```python
from build123d import *

# Parameters (mm, degrees)
F0_W      = 40
F0_H      = 11
F1_DEPTH  = 10
F2_R      = 8
F3_DEPTH  = 6
F4_R      = 6
F5_DEPTH  = 6
F6_W      = 11
F6_H      = 10
F7_DEPTH  = 2
F8_W      = 11
F8_H      = 10
F9_DEPTH  = 2
F10_R     = 5
F11_R     = 1.75
F12_DEPTH = 25
F13_R     = 2.75
F13_R_2   = 1.75
F14_DEPTH = 2


with BuildPart() as f1:
    # F0 (on Top) → F1 (new body)
    with BuildSketch(Plane.XY):
        with Locations((20, 5.5)):
            Rectangle(F0_W, F0_H)
    extrude(amount=F1_DEPTH)

    # F2 (on face) → F3 (cut)
    with BuildSketch(Plane.XZ):
        with Locations((20, 10)):
            Circle(F2_R)
    extrude(amount=-F3_DEPTH, mode=Mode.SUBTRACT)

    # F4 (on face) → F5 (cut)
    with BuildSketch(Plane(origin=(0, 11, 0), x_dir=(-1, 0, 0), z_dir=(0, 1, 0))):
        with Locations((-20, 10)):
            Circle(F4_R)
    extrude(amount=-F5_DEPTH, mode=Mode.SUBTRACT)

    # F6 (on face) → F7 (join)
    with BuildSketch(Plane(origin=(0, 0, 0), x_dir=(0, -1, 0), z_dir=(-1, 0, 0))):
        with Locations((-5.5, 5)):
            Rectangle(F6_W, F6_H)
    extrude(amount=F7_DEPTH)

    # F8 (on face) → F9 (join)
    with BuildSketch(Plane.YZ.offset(40)):
        with Locations((5.5, 5)):
            Rectangle(F8_W, F8_H)
    extrude(amount=F9_DEPTH)

    # F10
    f10_edges = [f1.edges().sort_by_distance(p)[0] for p in [
        (42, 11, 5),
        (42, 0, 5),
        (-2, 11, 5),
        (-2, 0, 5),
    ]]
    fillet(f10_edges, radius=F10_R)

    # F11 (on face) → F12 (cut)
    with BuildSketch(Plane.XY.offset(10)):
        with Locations((3.75, 6.25)):
            Circle(F11_R)
        with Locations((36.25, 6.25)):
            Circle(F11_R)
    extrude(amount=-F12_DEPTH, mode=Mode.SUBTRACT)

    # F13 (on face) → F14 (cut)
    with BuildSketch(Plane(origin=(0, 0, 0), x_dir=(1, 0, 0), z_dir=(0, 0, -1))):
        with Locations((3.75, -6.25)):
            Circle(F13_R)
        with Locations((3.75, -6.25)):
            Circle(F13_R_2, mode=Mode.SUBTRACT)
        with Locations((36.25, -6.25)):
            Circle(F13_R)
        with Locations((36.25, -6.25)):
            Circle(F13_R_2, mode=Mode.SUBTRACT)
    extrude(amount=-F14_DEPTH, mode=Mode.SUBTRACT)


solid = f1.part
```
CAD build for the part. Positions are in the model's coordinates, mm. A direction names the side the tool comes from. Coordinates: 2 decimals unless noted, no trailing zeros. Loops run counter-clockwise (first coordinate to the right, second up) from the corner with the lowest first, then second, coordinate; pieces in that order, holes last. Notation, with made-up numbers: (-9.75, 64) - (43.25, 64) arc R10 ccw to (43.25, 76) - close; hole circle Ø11 at (67.25, 24). An arc over 180 degrees is marked (long way). Return JSON: item names as keys, results as strings.
1. Mould opens along X. For faces 1 (the cylindrical face through (0, 10, 5)), 2 (the cylindrical face through (37.06, 4.7, 6.06)), 3 (the flat face through (38, 7, 2)), 4 (the flat face through (19.8, 11, 3.8)) say: released by +X, released by -X, zero draft, split by the parting line, or undercut.
Result:
{"face 1": "released by -X", "face 2": "undercut", "face 3": "undercut", "face 4": "zero draft"}
2. Band-saw the part on C-C (z = 8.5). Give the cut face in (x, y), and give its area (3 significant figures).
Result:
{"outline": "(-2, 5) arc R5 ccw to (3, 0) - (12.14, 0) - (12.14, 6) - (14.19, 6) - (14.19, 11) - (3, 11) arc R5 ccw to (-2, 6) - close; (25.81, 6) - (27.86, 6) - (27.86, 0) - (37, 0) arc R5 ccw to (42, 5) - (42, 6) arc R5 ccw to (37, 11) - (25.81, 11) - close; hole circle Ø3.5 at (3.75, 6.25); hole circle Ø3.5 at (36.25, 6.25)", "area": "291 mm2"}
3. Drop flat-ended pins along their axis: pin 1 (1.5 mm diameter, centred on y = 1, z = 7, fed in from +X); pin 2 (1.6 mm diameter, centred on x = 36.5, y = 5, fed in from -Z); pin 3 (4 mm diameter, centred on y = 9, z = 3, fed in from -X); pin 4 (2 mm diameter, centred on x = 3.75, y = 6.25, fed in from +Z). Give the stop position or say it passes through.
Result:
{"pin 1": "stops at x = 40.8", "pin 2": "stops at z = 2", "pin 3": "stops at x = -1.9", "pin 4": "passes through"}
4. 3-axis set-ups, long thin cutter, end or side, ignore diameter. For faces 5 (the cylindrical face through (20, 3, 2)), 6 (the cylindrical face through (40, 1, 5)), 7 (the cylindrical face through (3.154, 8.935, 0.986)): which of +Z, -Z, +X, -X, +Y, -Y reach the whole face in a straight line?
Result:
{"face 5": "+Z, -Y", "face 6": "+Z, -Z, +X, -Y", "face 7": "-Z"}
5. Band-saw the part on B-B (y = 7.25). Give the cut face in (x, z).
Result:
{"outline": "(-1.84, 0) - (1.19, 0) - (1.19, 2) - (2.31, 2) - (2.31, 10) - (-1.84, 10) - close; (5.19, 2) - (6.31, 2) - (6.31, 0) - (33.69, 0) - (33.69, 2) - (34.81, 2) - (34.81, 10) - (26, 10) arc R6 cw to (14, 10) - (5.19, 10) - close; (37.69, 2) - (38.81, 2) - (38.81, 0) - (41.84, 0) - (41.84, 10) - (37.69, 10) - close"}
6. Band-saw the part on A-A (x = 36.25). Give the cut face in (y, z), and give its area (3 significant figures).
Result:
{"outline": "(0, 0) - (3.5, 0) - (3.5, 2) - (4.5, 2) - (4.5, 10) - (0, 10) - close; (8, 2) - (9, 2) - (9, 0) - (11, 0) - (11, 10) - (8, 10) - close", "area": "71.0 mm2"}
7. Band-saw the part on D-D (x = 20). Give the cut face in (y, z).
Result:
{"outline": "(0, 0) - (11, 0) - (11, 4) - (6, 4) - (6, 2) - (0, 2) - close"}
8. Probe L1, parallel to X at y = 6.25, z = 0.4; L2, parallel to Y at x = 3.75, z = 1.6; L3, parallel to Y at x = 36.25, z = 5. List the from-to ranges inside material, lowest first. Write a range as from..to.
Result:
{"L1": "x = -1.99..1, 6.5..33.5, 39..41.99", "L2": "y = 0..3.5, 9..11", "L3": "y = 0..4.5, 8..11"}
